```python
from build123d import *

# Parameters (mm, degrees)
SKETCH_R  = 15.5
PAD_DEPTH = 6


with BuildPart() as sphere:
    # Sphere → Sphere (revolve)
    with BuildSketch(Plane(origin=(0, 0, 21), x_dir=(1, 0, 0), z_dir=(0, -1, 0))):
        with BuildLine():
            ThreePointArc((0, -20), (20, 0), (0, 20))
            Line((0, 20), (0, -20))
        make_face()
    revolve(axis=Axis((0, 0, 21), (0, 0, 1)))


with BuildPart() as cut:
    # Sketch → Pad (new body)
    with BuildSketch(Plane.XY):
        Circle(SKETCH_R)
    extrude(amount=PAD_DEPTH)

    # Cut: cut Sphere
    add(sphere.part, mode=Mode.SUBTRACT)


solid = cut.part
```
Source: CAD feature listing. Evaluate the final solid. Frame: model axes, mm. Give positions to 0.01 mm unless a question says otherwise; leave off trailing zeros. Order: outer loops, then holes, each group sorted by start corner. A loop starts at its lowest first (then second) coordinate and runs counter-clockwise, first axis right, second up. Notation, with made-up numbers: (33.25, 53) -> (65.25, 53) arc R20 cw to (65.25, 58) -> close; hole circle Ø6 at (-15.75, 40). An arc over 180 degrees is marked (long way). Use a Markdown table: item, result.
Q1. Section A-A (x = 0). Return the cut outline in (y, z).
A:
| item | result |
|---|---|
| outline | (-15.5, 0) -> (15.5, 0) -> (15.5, 6) -> (13.23, 6) arc R20 cw to (-13.23, 6) -> (-15.5, 6) -> close |
Q2. Section D-D (z = 1.45). Return the cut outline in (x, y).
A:
| item | result |
|---|---|
| outline | circle Ø31 at (0, 0); hole circle Ø8.44 at (0, 0) |
Q3. First-contact query: P1, Ø12, axis at x = -1.5, y = -2, coming from the +Z side; P2, Ø3, axis at x = -7, z = 3, coming from the -Y side; P3, Ø3, axis at x = -5.5, z = 3, coming from the +Y side (3 decimals). Flat tips, straight axial feed; report the tip coordinate or a pass-through.
A:
| item | result |
|---|---|
| P1 | z = 2.9 |
| P2 | y = -14.49 |
| P3 | y = 14.975 |
Q4. Section C-C (z = 5.05). Return the cut outline in (x, y), and give its area (3 significant figures).
A:
| item | result |
|---|---|
| outline | circle Ø31 at (0, 0); hole circle Ø24.13 at (0, 0) |
| area | 297 mm^2 |
Q5. Material intervals for line 1 (Y direction, x = -9, z = 5.75); line 2 (X direction, y = 8.5, z = 5.15); line 3 (Y direction, x = 1.5, z = 4.55), sorted ascending. Write a range as [from, to].
A:
| item | result |
|---|---|
| line 1 | [-12.62, -9.3], [9.3, 12.62] |
| line 2 | [-12.96, -8.75], [8.75, 12.96] |
| line 3 | [-15.43, -11.28], [11.28, 15.43] |
